Solid Edge part; units mm, degrees
sketch "Sketch1" plane through (0, 0, 0) normal (0, 0, 1) x (1, 0, 0)
  line L0 (0, 0) -> (0, 10)
  line L1 (0, 10) -> (4, 10)
  line L2 (4, 10) -> (4, 4)
  line L3 (4, 4) -> (10, 4)
  line L4 (10, 4) -> (10, 0)
  line L5 (10, 0) -> (0, 0)
  dimension "D1" = 10
  dimension "D2" = 10
extrude "Protrusion1" add sketch "Sketch1" along normal blind 113.5
sketch "Sketch2" plane through (5, 5, 113.5) normal (0, 0, 1) x (0, 1, 0)
  line L0 (5, 1) -> (5, 3)
  line L1 (5, 3) -> (-3, 3)
  line L2 (-3, 3) -> (-3, -5)
  line L3 (-3, -5) -> (-1, -5)
  line L4 (-1, -5) -> (-1, 1)
  line L5 (-1, 1) -> (5, 1)
extrude "ExtrudedCutout_4" cut sketch "Sketch2" against normal blind 5
sketch "Sketch3" plane through (5, 5, 0) normal (0, 0, -1) x (-1, 0, 0)
  line L0 (3, 5) -> (5, 5)
  line L1 (5, 5) -> (5, -5)
  line L2 (5, -5) -> (-5, -5)
  line L3 (-5, -5) -> (-5, -3)
  line L4 (-5, -3) -> (3, -3)
  line L5 (3, -3) -> (3, 5)
extrude "ExtrudedCutout_5" cut sketch "Sketch3" against normal blind 5
sketch "Sketch4" plane through (4, 6.5, 54.25) normal (1, 0, 0) x (0, 0, -1)
  line L0 (-52.5, 3.5) -> (-47.5, 3.5)
  line L1 (-47.5, 3.5) -> (-47.5, -2.5)
  line L2 (-47.5, -2.5) -> (-52.5, -2.5)
  line L3 (-52.5, -2.5) -> (-52.5, 3.5)
  dimension "D1" = 52.5
extrude "ExtrudedCutout_7" cut sketch "Sketch4" against normal blind 2
sketch "Sketch5" plane through (5.75, 4, 54.25) normal (0, 1, 0) x (0, 0, -1)
  line L0 (-52.5, 3.75) -> (-52.5, -4.25)
  line L1 (-52.5, -4.25) -> (-47.5, -4.25)
  line L2 (-47.5, -4.25) -> (-47.5, 3.75)
  line L3 (-47.5, 3.75) -> (-52.5, 3.75)
extrude "ExtrudedCutout_8" cut sketch "Sketch5" against normal blind 2
sketch "Sketch6" plane through (4, 6.5, 50.875) normal (1, 0, 0) x (0, 0, -1)
  line L0 (44.125, 3.5) -> (39.125, 3.5)
  line L1 (39.125, 3.5) -> (39.125, -2.5)
  line L2 (39.125, -2.5) -> (44.125, -2.5)
  line L3 (44.125, -2.5) -> (44.125, 3.5)
  dimension "D1" = 44.125
extrude "ExtrudedCutout_9" cut sketch "Sketch6" against normal blind 2
sketch "Sketch7" plane through (5.75, 4, 50.875) normal (0, 1, 0) x (0, 0, -1)
  line L0 (39.125, 3.75) -> (39.125, -4.25)
  line L1 (39.125, -4.25) -> (44.125, -4.25)
  line L2 (44.125, -4.25) -> (44.125, 3.75)
  line L3 (44.125, 3.75) -> (39.125, 3.75)
  dimension "D1" = 39.125
extrude "ExtrudedCutout_10" cut sketch "Sketch7" against normal blind 2
sketch "Sketch8" plane through (4, 7, 56.75) normal (1, 0, 0) x (0, 0, -1)
  circle A0 centre (-40, 0) radius 1.5
  circle A1 centre (-30, 0) radius 1.5
  circle A2 centre (-20, 0) radius 1.5
  circle A3 centre (-10, 0) radius 1.5
  circle A4 centre (0, 0) radius 1.5
  circle A5 centre (10, 0) radius 1.5
  circle A6 centre (20, 0) radius 1.5
  circle A7 centre (30, 0) radius 1.5
  circle A8 centre (40, 0) radius 1.5
extrude "ExtrudedCutout_11" cut sketch "Sketch8" against normal blind 4
sketch "Sketch9" plane through (7, 4, 56.75) normal (0, 1, 0) x (0, 0, 1)
  circle A0 centre (-40, 0) radius 1.5
  circle A1 centre (-30, 0) radius 1.5
  circle A2 centre (-20, 0) radius 1.5
  circle A3 centre (-10, 0) radius 1.5
  circle A4 centre (0, 0) radius 1.5
  circle A5 centre (10, 0) radius 1.5
  circle A6 centre (20, 0) radius 1.5
  circle A7 centre (30, 0) radius 1.5
  circle A8 centre (40, 0) radius 1.5
  dimension "D1" = 40
extrude "ExtrudedCutout_12" cut sketch "Sketch9" against normal blind 4
sketch "Sketch10" plane through (6, 4, 111) normal (0, 1, 0) x (-1, 0, 0)
  circle A0 centre (-1, -0.5) radius 1
  circle A1 centre (-1, -108) radius 1
  dimension "D1" = 1
extrude "ExtrudedCutout_13" cut sketch "Sketch10" against normal blind 4
sketch "Sketch11" plane through (4, 7, 3.375) normal (1, 0, 0) x (0, 1, 0)
  circle A0 centre (0, -0.375) radius 1
  circle A1 centre (0, 107.125) radius 1
extrude "ExtrudedCutout_14" cut sketch "Sketch11" against normal blind 4
sketch "Sketch12" plane through (6, 2, 9.25) normal (0, 1, 0) x (-1, 0, 0)
  circle A0 centre (-1, 0.5) radius 1
  circle A1 centre (-1, 95.5) radius 1
extrude "ExtrudedCutout_15" cut sketch "Sketch12" against normal blind 2
sketch "Sketch13" plane through (2, 6, 104.25) normal (1, 0, 0) x (0, 1, 0)
  circle A0 centre (1, -0.5) radius 1
  circle A1 centre (1, -95.5) radius 1
  dimension "D1" = 1
extrude "ExtrudedCutout_16" cut sketch "Sketch13" against normal blind 2
Check sheet for the modelled part. Datum: model origin and axes. Units: mm. A direction names the side the tool comes from. Round coordinates to 2 decimals unless told otherwise and drop trailing zeros. Loops run counter-clockwise (first coordinate to the right, second up) from the corner with the lowest first, then second, coordinate; pieces in that order, holes last. Notation, with made-up numbers: M -22,-15 L 9,-15 A11 ccw 9,-1 Z; hole C 31,65 d10. An arc over 180 degrees is marked long. One line per item, written item: value.
(1) Release check for a two-part mould opening along X. For faces 1 (the face through (0, 5, 58)), 2 (the face through (2, 5.9, 104.3)), 3 (the face through (6, 2, 9)), 4 (the face through (7, 3, 4)) record: +X half, -X half, draft (parallel to the pull), parting line (faces both ways), or undercut.
Computed values:
face 1: -X half
face 2: +X half
face 3: draft
face 4: undercut
(2) Sectioned sample at C-C, the plane x = 7. Count the separate pieces of the cut face and the enclosed holes in it, then the cut area to 3 significant figures.
Computed values:
separate pieces: 14
enclosed holes: 0
area: 290 mm^2
(3) Depth check by flat-ended pin: pin 1 Ø2.5 at (y, z) = (7, 66.75) entering from +X; pin 2 Ø5 at (y, z) = (8, 43.5) entering from +X; pin 3 Ø3 at (x, z) = (7, 3) entering from +Y; pin 4 Ø2.5 at (x, z) = (7, 9.75) entering from +Y. Enter the tip coordinate at first touch or a pass-through.
Computed values:
pin 1: passes through
pin 2: stops at x = 4
pin 3: stops at y = 4
pin 4: stops at y = 2
(4) Thickness scan on line 1 (X direction, y = 1, z = 57); line 2 (Y direction, x = 3.25, z = 76.75); line 3 (X direction, y = 9, z = 95). Record the ranges inside material, lowest first.
Computed values:
line 1: x = 0 to 5.52, 8.48 to 10
line 2: y = 0 to 5.5, 8.5 to 10
line 3: x = 0 to 4
(5) Sectioned sample at A-A, the plane z = 3. Record the cut outline in (x, y).
Computed values:
outline: M 2,2 L 6,2 L 6,4 L 4,4 L 4,6 L 2,6 Z; M 2,8 L 4,8 L 4,10 L 2,10 Z; M 8,2 L 10,2 L 10,4 L 8,4 Z
(6) Sectioned sample at B-B, the plane z = 110.5. Record the cut outline in (x, y).
Computed values:
outline: M 0,0 L 6,0 L 6,2 L 2,2 L 2,6 L 0,6 Z; M 0,8 L 2,8 L 2,10 L 0,10 Z; M 8,0 L 10,0 L 10,2 L 8,2 Z
(7) Access from +Z, -Z, +X, -X, +Y, -Y to the whole of each face (thin tool, end or side, straight path). Record for faces 5 (the face through (10, 2, 56)), 6 (the face through (6, 2, 104)), 7 (the face through (7, 4, 108)).
Computed values:
face 5: +Z, -Z, +X, +Y, -Y
face 6: +X, +Y
face 7: +Z, -Z, +X, +Y
(8) Sectioned sample at D-D, the plane z = 49.5. Record the cut outline in (x, y), then the cut area to 3 significant figures.
Computed values:
outline: M 0,0 L 10,0 L 10,4 L 4,4 L 4,10 L 0,10 Z
area: 64.0 mm^2
